```python
from build123d import *

# Parameters (mm, degrees)
ESQUISSE1_W             = 65
ESQUISSE1_H             = 85
BOSS_EXTRU_1_DEPTH      = 15
ESQUISSE2_W             = 58
ESQUISSE2_H             = 60
ENL_V_MAT_EXTRU_1_DEPTH = 11.5
ENL_V_MAT_EXTRU_2_DEPTH = 11.5
ESQUISSE5_W             = 12.942434053
ESQUISSE5_H             = 10
ENL_V_MAT_EXTRU_4_DEPTH = 81
ESQUISSE6_W             = 12.942434052
ESQUISSE6_H             = 10
ENL_V_MAT_EXTRU_5_DEPTH = 81
ESQUISSE7_W             = 9.561184164
ESQUISSE7_H             = 4.914624062
ENL_V_MAT_EXTRU_6_DEPTH = 81
ESQUISSE9_W             = 27
ESQUISSE9_H             = 15
BOSS_EXTRU_3_DEPTH      = 4
ENL_V_MAT_EXTRU_8_DEPTH = 4
ESQUISSE13_R            = 5
ESQUISSE13_W            = 2.4
ESQUISSE13_H            = 6.4
ENL_V_MAT_EXTRU_9_DEPTH = 4


with BuildPart() as part:
    # Esquisse1 → Boss.-Extru.1 (new body)
    with BuildSketch(Plane.XY):
        with Locations((-47.785104755, -14.386514523)):
            Rectangle(ESQUISSE1_W, ESQUISSE1_H)
    extrude(amount=BOSS_EXTRU_1_DEPTH)

    # Esquisse2 → Enlèv. mat.-Extru.1 (cut)
    with BuildSketch(Plane.XY.offset(15)):
        with Locations((-47.785104755, -14.828948576)):
            Rectangle(ESQUISSE2_W, ESQUISSE2_H)
    extrude(amount=-ENL_V_MAT_EXTRU_1_DEPTH, mode=Mode.SUBTRACT)

    # Esquisse3 → Enlèv. mat.-Extru.2 (cut)
    with BuildSketch(Plane.XY.offset(15)):
        with BuildLine():
            Line((-31.727538807, 28.113485477), (-63.842670702, 28.113485477))
            ThreePointArc((-63.842670702, 28.113485477), (-67.633421871, 18.961802593), (-76.785104755, 15.171051424))
            Line((-76.785104755, 15.171051424), (-18.785104755, 15.171051424))
            ThreePointArc((-18.785104755, 15.171051424), (-27.936787638, 18.961802593), (-31.727538807, 28.113485477))
        make_face()
        with BuildLine():
            ThreePointArc((-18.785104755, -44.828948576), (-24.482664276, -47.188955002), (-26.842670702, -52.886514523))
            Line((-26.842670702, -52.886514523), (-68.727538807, -52.886514523))
            ThreePointArc((-68.727538807, -52.886514523), (-71.087545234, -47.188955002), (-76.785104755, -44.828948576))
            Line((-76.785104755, -44.828948576), (-18.785104755, -44.828948576))
        make_face()
    extrude(amount=-ENL_V_MAT_EXTRU_2_DEPTH, mode=Mode.SUBTRACT)

    # Esquisse5 → Enlèv. mat.-Extru.4 (cut)
    with BuildSketch(Plane(origin=(0, 28.113485477, 0), x_dir=(1, 0, 0), z_dir=(0, 1, 0))):
        with Locations((-70.313887729, -8.5)):
            Rectangle(ESQUISSE5_W, ESQUISSE5_H)
    extrude(amount=-ENL_V_MAT_EXTRU_4_DEPTH, mode=Mode.SUBTRACT)

    # Esquisse6 → Enlèv. mat.-Extru.5 (cut)
    with BuildSketch(Plane(origin=(0, 28.113485477, 0), x_dir=(1, 0, 0), z_dir=(0, 1, 0))):
        with Locations((-25.256321781, -8.5)):
            Rectangle(ESQUISSE6_W, ESQUISSE6_H)
    extrude(amount=-ENL_V_MAT_EXTRU_5_DEPTH, mode=Mode.SUBTRACT)

    # Esquisse7 → Enlèv. mat.-Extru.6 (cut)
    with BuildSketch(Plane(origin=(0, -56.886514523, 0), x_dir=(-1, 0, 0), z_dir=(0, -1, 0))):
        with Locations((47.785104755, -7.5)):
            Rectangle(ESQUISSE7_W, ESQUISSE7_H)
    extrude(amount=-ENL_V_MAT_EXTRU_6_DEPTH, mode=Mode.SUBTRACT)

    # Esquisse9 → Boss.-Extru.3 (add)
    with BuildSketch(Plane(origin=(0, 0, 0), x_dir=(-1, 0, 0), z_dir=(0, 0, -1))):
        with Locations((47.785104755, 7.665180304)):
            Rectangle(ESQUISSE9_W, ESQUISSE9_H)
    extrude(amount=BOSS_EXTRU_3_DEPTH)

    # Esquisse10 → Enlèv. mat.-Extru.8 (cut)
    with BuildSketch(Plane(origin=(0, 0, -4), x_dir=(-1, 0, 0), z_dir=(0, 0, -1))):
        Polygon((42.785104755, 15.165180304), (44.785104755, 6.365180304), (36.285104755, 6.365180304), (38.285104755, 15.165180304), align=None)
        Polygon((52.785104755, 15.165180304), (50.785104755, 6.365180304), (59.285104755, 6.365180304), (57.285104755, 15.165180304), align=None)
    extrude(amount=-ENL_V_MAT_EXTRU_8_DEPTH, mode=Mode.SUBTRACT)

    # Esquisse13 → Enlèv. mat.-Extru.9 (cut)
    with BuildSketch(Plane(origin=(-15.285104755, 0, 0), x_dir=(0, 0, -1), z_dir=(1, 0, 0))):
        with Locations((-9.118338435, 14.613485477)):
            Circle(ESQUISSE13_R)
        with Locations((-9.118338435, -43.386514523)):
            Circle(ESQUISSE13_R)
        with Locations((-9.218338435, 17.790714068)):
            Rectangle(ESQUISSE13_W, ESQUISSE13_H)
        with Locations((-9.218338435, -40.186514523)):
            Rectangle(ESQUISSE13_W, ESQUISSE13_H)
    extrude(amount=-ENL_V_MAT_EXTRU_9_DEPTH, mode=Mode.SUBTRACT)


solid = part.part
```
Input: part model. Units: mm. Frame: model coordinates. A direction names the side the tool comes from. Coordinates: 2 decimals unless noted, no trailing zeros. Loops run counter-clockwise (first coordinate to the right, second up) from the corner with the lowest first, then second, coordinate; pieces in that order, holes last. Notation, with made-up numbers: M 52.25,-34 L 76.25,-34 A16 ccw 76.25,-11 Z; hole C -1,27 d1. An arc over 180 degrees is marked long. Use a Markdown table: item, result. Add a question column.
1) Section A-A, the plane x = -28. Return the cut outline in (y, z).
2) Section B-B, the plane z = 7. Return the cut outline in (x, y), plus the area to 3 significant figures.
3) Pin query (flat end, axial travel): P1, Ø0.5, axis at x = -17, y = -37.5, coming from the -Z side; P2, Ø10, axis at y = 17, z = 7.5, coming from the +X side; P3, Ø2, axis at x = -61.5, y = -35.5, coming from the +Z side; P4, Ø2, axis at x = -60.5, z = -2.5, coming from the +Y side. Return the tip coordinate at first contact, or that it passes through.
4) Draft query along X for faces 6 (the flat face through (-22, -50, 13.5)), 7 (the flat face through (-48, 6, -4)), 8 (the flat face through (-80.285, -15, 7)), 9 (the flat face through (-34.285, 8, -2)). Return one class per face: +X half, -X half, draft (parallel to the pull), parting line (faces both ways), or undercut.
5) Section D-D, the plane z = 11.5. Return the cut outline in (x, y), plus the area to 3 significant figures.
6) Set-up query: faces 1 (the cylindrical face through (-17.257, -48.386, 9.218)), 2 (the flat face through (-24, 23, 13.5)), 3 (the flat face through (-36, 15.165, -2)), 4 (the flat face through (-61.285, 8, -2)), 5 (the flat face through (-48, 0.165, -2)). Return all of +Z, -Z, +X, -X, +Y, -Y with unobstructed straight access to the full face (end or side cutting, diameter ignored); none if empty.
7) Section C-C, the plane y = -17.5. Return the cut outline in (x, z).
8) Line query: L1, parallel to X at y = 22, z = 5.25; L2, parallel to Z at x = -66, y = 21.5; L3, parallel to Z at x = -26.5, y = -16.5. Output: solid intervals per line, ascending. Write a range as from..to.
Answer below:
| question | item | result |
|---|---|---|
| 1 | outline | M -56.89,0 L 28.11,0 L 28.11,3.5 L -52.89,3.5 L -52.89,15 L -56.89,15 Z; M 19.03,13.5 L 28.11,13.5 L 28.11,15 L 19.03,15 Z |
| 2 | outline | M -80.29,-56.89 L -52.57,-56.89 L -52.57,-52.89 L -76.79,-52.89 L -76.79,28.11 L -80.29,28.11 Z; M -43,-56.89 L -15.29,-56.89 L -15.29,-47.92 L -18.79,-47.92 L -18.79,-52.89 L -43,-52.89 Z; M -18.79,-38.86 L -15.29,-38.86 L -15.29,10.08 L -18.79,10.08 Z; M -18.79,19.14 L -15.29,19.14 L -15.29,28.11 L -18.79,28.11 Z |
| 2 | area | 725 mm2 |
| 3 | P1 | z = 0 |
| 3 | P2 | x = -15.29 |
| 3 | P3 | z = 3.5 |
| 3 | P4 | y = 15.17 |
| 4 | face 6 | undercut |
| 4 | face 7 | draft |
| 4 | face 8 | -X half |
| 4 | face 9 | +X half |
| 5 | outline | M -80.29,-56.89 L -15.29,-56.89 L -15.29,-47.78 L -18.79,-47.78 L -18.79,-52.89 L -76.79,-52.89 L -76.79,28.11 L -80.29,28.11 Z; M -18.79,-38.99 L -15.29,-38.99 L -15.29,10.22 L -18.79,10.22 Z; M -18.79,19.01 L -15.29,19.01 L -15.29,28.11 L -18.79,28.11 Z |
| 5 | area | 765 mm2 |
| 6 | face 1 | +X |
| 6 | face 2 | +Y |
| 6 | face 3 | -Z, +X, -X, +Y |
| 6 | face 4 | -Z, -X, +Y, -Y |
| 6 | face 5 | -Z, +X, -X, -Y |
| 7 | outline | M -80.29,0 L -15.29,0 L -15.29,15 L -18.79,15 L -18.79,3.5 L -76.79,3.5 L -76.79,15 L -80.29,15 Z |
| 8 | L1 | -80.29..-76.79, -18.79..-15.29 |
| 8 | L2 | 0..3.5, 13.5..15 |
| 8 | L3 | 0..3.5 |
